Part model, mm, in its own coordinate system. A direction names the side the tool comes from. Coordinates: 2 decimals unless noted, no trailing zeros. Loops run counter-clockwise (first coordinate to the right, second up) from the corner with the lowest first, then second, coordinate; pieces in that order, holes last. Notation, with made-up numbers: (27.5, 47) - (73.5, 47) arc R29 cw to (73.5, 83) - close; hole circle Ø11 at (30.5, 7.5). An arc over 180 degrees is marked (long way). Use a Markdown table: item, result. Add a question column.
1. 3-axis set-ups, long thin cutter, end or side, ignore diameter. For faces 1 (the flat face through (0, 0, 0)), 2 (the cylindrical face through (0, 5, 8)), 3 (the cylindrical face through (0.34, 32.78, 1.55)): which of +Z, -Z, +X, -X, +Y, -Y reach the whole face in a straight line?
2. Band-saw the part on B-B, the plane y = 20. Give the cut face in (x, z), plus the area to 3 significant figures.
3. Band-saw the part on A-A, the plane y = 7. Give the cut face in (x, z).
4. Band-saw the part on C-C, the plane y = 26. Give the cut face in (x, z).
5. Wall check: probe 1 along Z at (x, y) = (0, 4.75); probe 2 along Y at (x, z) = (-7.75, -2.75); probe 3 along X at (y, z) = (15, 0.25). Give the ranges that are in metal, low to high. Write a range as [from, to].
6. Drop flat-ended pins along their axis: pin 1 (8 mm diameter, centred on y = 7.5, z = 10.5, fed in from +X); pin 2 (0.9 mm diameter, centred on x = 0.5, z = -9.5, fed in from -Y); pin 3 (14 mm diameter, centred on x = -4, z = 6.5, fed in from -Y); pin 4 (4 mm diameter, centred on x = 9.5, z = 0, fed in from +Y). Give the stop position or say it passes through.
7. Pull direction X, two halves, no side cores. Call faces 4 (the cylindrical face through (0, 5, -11)), 5 (the flat face through (0, 25, -8.2)), 6 (the cylindrical face through (3, 12.63, 13.52)): pulls with the +X half, pulls with the -X half, needs draft (parallel to the pull), parting line crosses it, or undercut.
from build123d import *

# Parameters (mm, degrees)
SKETCH3_R          = 1.5
CUT_EXTRUDE1_DEPTH = 10


with BuildPart() as part:
    # Sketch2 → Revolve1 (revolve)
    with BuildSketch(Plane.XY, mode=Mode.PRIVATE) as revolve1_sk:
        Polygon((0, 0), (11, 0), (12.732050808, 3), (13.85, 3), (13.85, 22), (10, 25), (8, 25), (8, 27), (1.585, 27), (1.585, 38.4), (0, 38.4), align=None)
    revolve(revolve1_sk.sketch.rotate(Axis((0, 38.4, 0), (0, -1, 0)), 180), axis=Axis((0, 38.4, 0), (0, -1, 0)))

    # Sketch3 → Cut-Extrude1 (cut)
    with BuildSketch(Plane.XZ):
        with Locations((9.5, 0)):
            Circle(SKETCH3_R)
        with Locations((-8, 0)):
            Circle(SKETCH3_R)
        with Locations((0, 9.5)):
            Circle(SKETCH3_R)
        with Locations((0, -9.5)):
            Circle(SKETCH3_R)
    extrude(amount=-CUT_EXTRUDE1_DEPTH, mode=Mode.SUBTRACT)


solid = part.part
Geometry check:
| question | item | result |
|---|---|---|
| 1 | face 1 | +Z, -Z, +X, -X, -Y |
| 1 | face 2 | -Y |
| 1 | face 3 | +Y |
| 2 | outline | circle Ø27.7 at (0, 0) |
| 2 | area | 603 mm^2 |
| 3 | outline | circle Ø27.7 at (0, 0); hole circle Ø3 at (-8, 0); hole circle Ø3 at (0, -9.5); hole circle Ø3 at (0, 9.5); hole circle Ø3 at (9.5, 0) |
| 4 | outline | circle Ø16 at (0, 0) |
| 5 | probe 1 | z = [-13.85, -11], [-8, 8], [11, 13.85] |
| 5 | probe 2 | y = [0, 25] |
| 5 | probe 3 | x = [-13.85, 13.85] |
| 6 | pin 1 | stops at x = 12.23 |
| 6 | pin 2 | stops at y = 10 |
| 6 | pin 3 | stops at y = 0 |
| 6 | pin 4 | stops at y = 27 |
| 7 | face 4 | undercut |
| 7 | face 5 | needs draft |
| 7 | face 6 | parting line crosses it |
